Verification items for the finished model (mm, model axes). A direction names the side the tool comes from. Give positions to 0.01 mm unless a question says otherwise; leave off trailing zeros. Order: outer loops, then holes, each group sorted by start corner. A loop starts at its lowest first (then second) coordinate and runs counter-clockwise, first axis right, second up. Notation, with made-up numbers: (85.5, 14.25) - (89.5, 14.25) arc R14 ccw to (89.5, 22.25) - close; hole circle Ø6 at (60, 62.25). An arc over 180 degrees is marked (long way). Answer as a JSON object with one key per item and string values.
```python
from build123d import *

# Parameters (mm, degrees)
F1_DEPTH = 7.05
F2_COUNT = 3


with BuildPart() as f1:
    # F0 (on Top) → F1 (new body)
    with BuildSketch(Plane.XY):
        with BuildLine():
            ThreePointArc((10, 43.9972005226), (-0.6298612389, 53.9773445506), (-9.9206549639, 42.7399793461))
            Line((-9.9206549639, 42.7399793461), (-9.9206549639, 43.9972005226))
            Line((-9.9206549639, 43.9972005226), (-6.3003222272, 43.9972005226))
            Line((-6.3003222272, 43.9972005226), (-6.2644989641, 47.6981147533))
            Line((-6.2644989641, 47.6981147533), (0.0704118404, 51.2742726216))
            Line((0.0704118404, 51.2742726216), (6.3349108045, 47.5761578682))
            Line((6.3349108045, 47.5761578682), (6.3002680318, 43.9972005226))
            Line((6.3002680318, 43.9972005226), (10, 43.9972005226))
        make_face()
        with BuildLine():
            Line((-9.9206549639, 43.9972005226), (-9.9206549639, 42.7399793461))
            ThreePointArc((-9.9206549639, 42.7399793461), (0.6298612389, 34.0170564946), (10, 43.9972005226))
            Line((10, 43.9972005226), (6.3002680318, 43.9972005226))
            Line((6.3002680318, 43.9972005226), (6.2644989641, 40.3018852467))
            Line((6.2644989641, 40.3018852467), (-0.0704118404, 36.7257273784))
            Line((-0.0704118404, 36.7257273784), (-6.3349108045, 40.4238421318))
            Line((-6.3349108045, 40.4238421318), (-6.3003222272, 43.9972005226))
            Line((-6.3003222272, 43.9972005226), (-9.9206549639, 43.9972005226))
        make_face()
        with BuildLine():
            ThreePointArc((-9.9206549639, 9.878289583), (0.1133775368, 13.9995409044), (10.0793450361, 9.7163163619))
            Line((10.0793450361, 9.7163163619), (10.0793450361, 43.9972005226))
            Line((10.0793450361, 43.9972005226), (10, 43.9972005226))
            ThreePointArc((10, 43.9972005226), (0.6298612389, 34.0170564946), (-9.9206549639, 42.7399793461))
            Line((-9.9206549639, 42.7399793461), (-9.9206549639, 9.878289583))
        make_face()
        Polygon((6.4861108845, 28.5761578682), (6.415699044, 21.3018852467), (0.0807882395, 17.7257273784), (-6.1837107246, 21.4238421318), (-6.1132988842, 28.6981147533), (0.2216119204, 32.2742726216), align=None, mode=Mode.SUBTRACT)
        with BuildLine():
            ThreePointArc((6.3718920076, 8.9972005226), (9.7928732858, 5.0646083568), (11.025, 0))
            ThreePointArc((11.025, 0), (-5.0646083568, -9.7928732858), (-6.3718920076, 8.9972005226))
            Line((-6.3718920076, 8.9972005226), (-9.9206549639, 8.9972005226))
            Line((-9.9206549639, 8.9972005226), (-9.9206549639, 9.878289583))
            ThreePointArc((-9.9206549639, 9.878289583), (-5.3437267195, -12.9400380505), (14, 0))
            ThreePointArc((14, 0), (12.982889326, 5.2387579394), (10.0793450361, 9.7163163619))
            Line((10.0793450361, 9.7163163619), (10.0793450361, 8.9972005226))
            Line((10.0793450361, 8.9972005226), (6.3718920076, 8.9972005226))
        make_face()
        with BuildLine():
            ThreePointArc((-6.3718920076, 8.9972005226), (0, 11.025), (6.3718920076, 8.9972005226))
            Line((6.3718920076, 8.9972005226), (10.0793450361, 8.9972005226))
            Line((10.0793450361, 8.9972005226), (10.0793450361, 9.7163163619))
            ThreePointArc((10.0793450361, 9.7163163619), (0.1133775368, 13.9995409044), (-9.9206549639, 9.878289583))
            Line((-9.9206549639, 9.878289583), (-9.9206549639, 8.9972005226))
            Line((-9.9206549639, 8.9972005226), (-6.3718920076, 8.9972005226))
        make_face()
    extrude(amount=F1_DEPTH)

    # F2: F1 ×3 about axis
    f2_axis = Axis((0, 0, 0), (0, 0, -1))


with BuildPart() as f1_1:
    add(f1.part)
    for i in range(1, F2_COUNT):
        add(f1.part.rotate(f2_axis, i * 360 / F2_COUNT))


solid = f1_1.part
```
(1) Release check for a two-part mould opening along Y. For faces 3 (the flat face through (34.96, -16.54, 3.48)), 4 (the flat face through (-18.02, -21.86, 3.48)), 5 (the flat face through (-28.09, -4.58, 3.48)) record: pulls with the +Y half, pulls with the -Y half, needs draft (parallel to the pull), parting line crosses it, or undercut.
Computed values:
{"face 3": "undercut", "face 4": "pulls with the -Y half", "face 5": "pulls with the +Y half"}
(2) Section check A-A (x = 36). Record the cut outline in (y, z).
Computed values:
{"outline": "(-31.78, 0) - (-28.07, 0) - (-28.07, 7.05) - (-31.78, 7.05) - close; (-15.95, 0) - (-9.33, 0) - (-9.33, 7.05) - (-15.95, 7.05) - close"}
(3) Section check B-B (z = 4.25). Count the separate pieces of the cut face and the enclosed holes in it, then the cut area to 3 significant figures.
Computed values:
{"separate pieces": "1", "enclosed holes": "7", "area": "1,760 mm²"}
(4) Material ranges on line 1 along X through (y, z) = (-22, 5.75); line 2 along Y through (x, z) = (-5.5, 1.75); line 3 along X through (y, z) = (-18.5, 2.25), recorded low to high. Write a range as [from, to].
Computed values:
{"line 1": "x = [-48.1, -44.41], [-31.8, -18.26], [17.95, 31.8], [44.41, 48.1]", "line 2": "y = [-14.63, -9.56], [9.56, 21.02], [29.04, 39.93], [48.13, 52.35]", "line 3": "x = [-47.47, -44.37], [-31.77, -23.73], [-19.77, -12.2], [11.88, 19.12], [23.99, 31.84], [44.44, 47.47]"}
(5) Access from +Z, -Z, +X, -X, +Y, -Y to the whole of each face (thin tool, end or side, straight path). Record for faces 1 (the flat face through (24.7, -18.1, 3.5)), 2 (the flat face through (27.944, -4.678, 3.476)).
Computed values:
{"face 1": "+Z, -Z", "face 2": "+Z, -Z, +X, +Y"}
(6) Gauge pin test, flat ends, axial feed: pin 1 Ø3.5 at (y, z) = (32.5, 5) entering from -X; pin 2 Ø1.5 at (y, z) = (3, 3.5) entering from +X. Record the tip position at first contact, or that the pin passes through.
Computed values:
{"pin 1": "stops at x = -9.92", "pin 2": "stops at x = 15.94"}
